Autodesk Inventor part; units mm, degrees
ref_plane "YZ Plane" through (0, 0, 0) normal (1, 0, 0) x (0, 1, 0)
ref_plane "XZ Plane" through (0, 0, 0) normal (0, 1, 0) x (-1, 0, 0)
ref_plane "XY Plane" through (0, 0, 0) normal (0, 0, 1) x (1, 0, 0)
sketch "Sketch1" plane through (0, 0, 0) normal (0, 0, 1) x (1, 0, 0)
  line L0 (6.25, -11.75) -> (-6.25, -11.75)
  line L1 (-6.25, -11.75) -> (-6.25, 11.75)
  line L2 (-6.25, 11.75) -> (6.25, 11.75)
  line L3 (6.25, 11.75) -> (6.25, -11.75)
  line L4 (6.25, -11.75) -> (-6.25, 11.75) construction
  line L5 (-6.25, -11.75) -> (6.25, 11.75) construction
  line L6 (9.25, 6.25) -> (-9.25, 6.25)
  line L7 (-9.25, 6.25) -> (-9.25, -6.25)
  line L8 (-9.25, -6.25) -> (9.25, -6.25)
  line L9 (9.25, -6.25) -> (9.25, 6.25)
  line L10 (9.25, 6.25) -> (-9.25, -6.25) construction
  line L11 (-9.25, 6.25) -> (9.25, -6.25) construction
  line L12 (-10.5, 16.75) -> (10.5, 16.75)
  line L13 (12.5, 14.75) -> (12.5, -24.75)
  line L14 (10.5, -26.75) -> (-10.5, -26.75)
  line L15 (-12.5, -24.75) -> (-12.5, 14.75)
  line L16 (-9, -13.5) -> (9, -13.5) construction
  line L17 (9, -13.5) -> (9, -23.5) construction
  line L18 (9, -23.5) -> (-9, -23.5) construction
  line L19 (-9, -23.5) -> (-9, -13.5) construction
  circle A0 centre (-9, -23.5) radius 1.75
  circle A1 centre (-9, -13.5) radius 1.75
  circle A2 centre (9, -13.5) radius 1.75
  circle A3 centre (9, -23.5) radius 1.75
  line L20 (-9, 13.5) -> (9, 13.5) construction
  circle A4 centre (-9, 13.5) radius 1.75
  circle A5 centre (9, 13.5) radius 1.75
  arc A6 (-10.5, 16.75) -> (-12.5, 14.75) centre (-10.5, 14.75) ccw
  arc A7 (12.5, 14.75) -> (10.5, 16.75) centre (10.5, 14.75) ccw
  arc A8 (10.5, -26.75) -> (12.5, -24.75) centre (10.5, -24.75) ccw
  arc A9 (-12.5, -24.75) -> (-10.5, -26.75) centre (-10.5, -24.75) ccw
  point P0 (0, 0)
  point P1 (-12.5, 16.75)
  point P2 (12.5, 16.75)
  point P3 (-12.5, -26.75)
  point P4 (0, 16.75)
  point P5 (0, 0)
  point P6 (0, -23.5)
  point P7 (0, 0)
  dimension "d0" = 43.5
  dimension "d1" = 25
  dimension "d2" = 23.5
  dimension "d3" = 12.5
  dimension "d4" = 18.5
  dimension "d5" = 12.5
  dimension "d6" = 16.75
  dimension "d7" = 18
  dimension "d8" = 10
  dimension "d9" = 3.5
  dimension "d10" = 3.25
  dimension "d11" = 3.25
  dimension "d12" = 2
extrude "Extrusion1" add sketch "Sketch1" against normal blind 2.8
Design review of the part built by this model. Coordinates are the model's own, in mm. A direction names the side the tool comes from. Round coordinates to 2 decimals unless told otherwise and drop trailing zeros. Write each loop counter-clockwise with the first axis right and the second up, starting at its lowest first coordinate (ties: lowest second). Pieces come first, ordered by that corner, then holes. Notation, with made-up numbers: (-6, 16.5) -> (35, 16.5) arc R25 ccw to (35, 44.5) -> close; hole circle Ø6 at (75.5, 31). An arc over 180 degrees is marked (long way). One line per item, written item: value. Start each with the question number.
Q1. Add section A-A (y = 9). Give the boundary of the cut face in (x, z).
Q2. Add section C-C (z = -1.75). Give the boundary of the cut face in (x, y).
Q3. The part is to be moulded in two halves that separate along Y. For faces 1 (the face through (0, 16.75, -1)), 2 (the face through (-12.5, -5, -1)), 3 (the face through (8, 6.25, -1)), say which applies: pulls with the +Y half, pulls with the -Y half, needs draft (parallel to the pull), parting line crosses it, or undercut.
Q4. To check wall thickness, follow probe 1 along Y at (x, z) = (-9, -1.35); probe 2 along X at (y, z) = (-10, -0.45); probe 3 along X at (y, z) = (-3.5, -1.85). State the ranges of each line that lie inside material, in increasing order.
Q5. Tool access review of faces 4 (the face through (12.5, -5, -1)), 5 (the face through (-6.25, -9, -1)): name each direction out of +Z, -Z, +X, -X, +Y, -Y from which nothing blocks a thin tool from reaching the whole face with its end or side.
Q6. Add section B-B (x = 2.5). Give the boundary of the cut face in (y, z), then the cut area to 3 significant figures.
Q7. Add section D-D (y = -23.5). Give the boundary of the cut face in (x, z), then the cut area to 3 significant figures.
Q8. Insertion check: P1, Ø3, axis at x = 9, y = 13.5, coming from the +Z side. The pin has a flat end and moves straight along its axis. Give the tip position at first contact, or say it passes through.
Response:
1. outline: (-12.5, -2.8) -> (-6.25, -2.8) -> (-6.25, 0) -> (-12.5, 0) -> close; (6.25, -2.8) -> (12.5, -2.8) -> (12.5, 0) -> (6.25, 0) -> close
2. outline: (-12.5, -24.75) arc R2 ccw to (-10.5, -26.75) -> (10.5, -26.75) arc R2 ccw to (12.5, -24.75) -> (12.5, 14.75) arc R2 ccw to (10.5, 16.75) -> (-10.5, 16.75) arc R2 ccw to (-12.5, 14.75) -> close; hole circle Ø3.5 at (-9, -23.5); hole circle Ø3.5 at (-9, -13.5); hole circle Ø3.5 at (-9, 13.5); hole (-9.25, -6.25) -> (-6.25, -6.25) -> (-6.25, -11.75) -> (6.25, -11.75) -> (6.25, -6.25) -> (9.25, -6.25) -> (9.25, 6.25) -> (6.25, 6.25) -> (6.25, 11.75) -> (-6.25, 11.75) -> (-6.25, 6.25) -> (-9.25, 6.25) -> close; hole circle Ø3.5 at (9, -23.5); hole circle Ø3.5 at (9, -13.5); hole circle Ø3.5 at (9, 13.5)
3. face 1: pulls with the +Y half
3. face 2: needs draft
3. face 3: undercut
4. probe 1: y = -26.75 to -25.25, -21.75 to -15.25, -11.75 to -6.25, 6.25 to 11.75, 15.25 to 16.75
4. probe 2: x = -12.5 to -6.25, 6.25 to 12.5
4. probe 3: x = -12.5 to -9.25, 9.25 to 12.5
5. face 4: +Z, -Z, +X, +Y, -Y
5. face 5: +Z, -Z
6. outline: (-26.75, -2.8) -> (-11.75, -2.8) -> (-11.75, 0) -> (-26.75, 0) -> close; (11.75, -2.8) -> (16.75, -2.8) -> (16.75, 0) -> (11.75, 0) -> close
6. area: 56.0 mm^2
7. outline: (-12.5, -2.8) -> (-10.75, -2.8) -> (-10.75, 0) -> (-12.5, 0) -> close; (-7.25, -2.8) -> (7.25, -2.8) -> (7.25, 0) -> (-7.25, 0) -> close; (10.75, -2.8) -> (12.5, -2.8) -> (12.5, 0) -> (10.75, 0) -> close
7. area: 50.4 mm^2
8. P1: passes through
